from build123d import *

# Parameters (mm, degrees)
SKETCH1_W = 6.35
SKETCH1_H = 7.9375
FILLET1_R = 0.79375


with BuildPart() as part:
    # Sketch1 → Revolve1 (revolve)
    with BuildSketch(Plane.XY, mode=Mode.PRIVATE) as revolve1_sk:
        with Locations((0, 10.31875)):
            Rectangle(SKETCH1_W, SKETCH1_H)
    revolve(revolve1_sk.sketch.rotate(Axis((0, 0, 0), (-1, 0, 0)), 90), axis=Axis((0, 0, 0), (-1, 0, 0)))

    # Fillet1
    fillet1_edges = [part.edges().sort_by_distance(p)[0] for p in [
        (-3.175, 0, 14.2875),
        (3.175, 0, 14.2875),
        (3.175, 0, 6.35),
        (-3.175, 0, 6.35),
    ]]
    fillet(fillet1_edges, radius=FILLET1_R)


solid = part.part
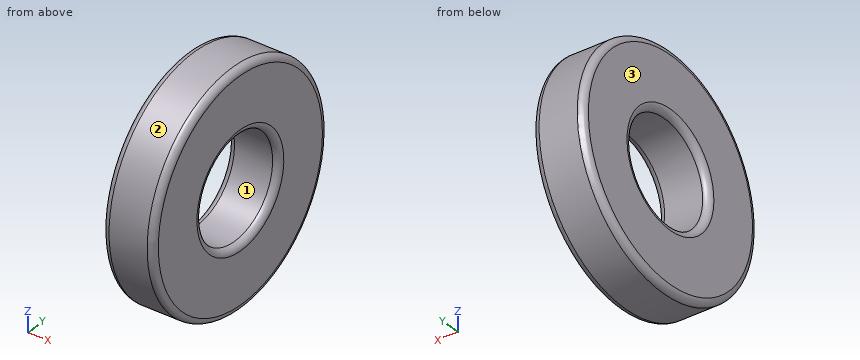
Geometry check sheet. Reference: the model listing, model coordinates, mm. Face numbers are marked on the shaded views. Give positions to 0.01 mm unless a question says otherwise; leave off trailing zeros. Write each question's results on one line, items separated by ' | '.
1) Gauge pin test, flat ends, axial feed: pin 1 (2 mm diameter, centred on x = -0.5, z = -5.5, fed in from -Y); pin 2 (2 mm diameter, centred on y = 0, z = 6, fed in from -X); pin 3 (3 mm diameter, centred on y = 1.5, z = -4, fed in from -X). Record the tip position at first contact, or that the pin passes through.
Answers follow:
pin 1: y = -13.56 | pin 2: x = -3.16 | pin 3: through
2) Thickness scan on line 1 (Y direction, x = 0.7, z = 0); line 2 (Z direction, x = -2, y = 4.75); line 3 (Z direction, x = 1.5, y = -5.25). Record the ranges inside material, lowest first.
Answers follow:
line 1: -14.29 to -6.35, 6.35 to 14.29 | line 2: -13.47 to -4.21, 4.21 to 13.47 | line 3: -13.29 to -3.57, 3.57 to 13.29
3) Release check for a two-part mould opening along Y. For the marked faces 1, 2 and 3 record: +Y half, -Y half, draft (parallel to the pull), parting line (faces both ways), or undercut.
Answers follow:
face 1: undercut | face 2: parting line | face 3: draft
